Source: CAD feature listing. Evaluate the final solid. Frame: model axes, mm. Face numbers are marked on the shaded views. Round coordinates to 2 decimals unless told otherwise and drop trailing zeros. Write each loop counter-clockwise with the first axis right and the second up, starting at its lowest first coordinate (ties: lowest second). Pieces come first, ordered by that corner, then holes. Notation, with made-up numbers: M 89.25,0.25 L 126.25,0.25 A7 cw 126.25,4.25 Z; hole C 34,71.25 d10. An arc over 180 degrees is marked long. Answer in a Markdown table with one row per item.
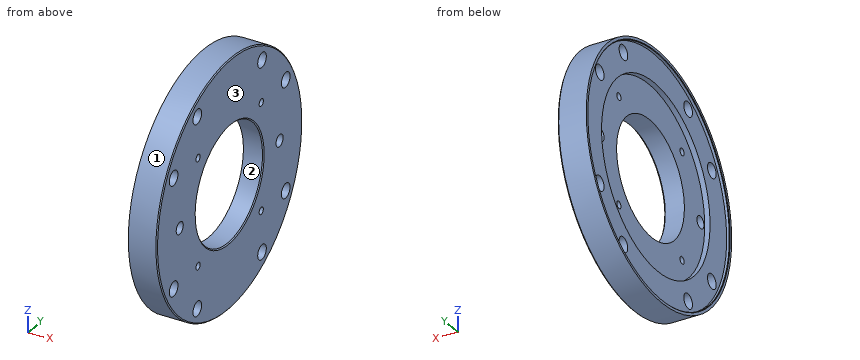
from build123d import *

# Parameters (mm, degrees)
CUT_EXTRUDE_1_DEPTH      = 170.04733065
CUT_EXTRUDE_1_DEPTH_BACK = 170.04733065
SKETCH_2_R               = 7
CUT_EXTRUDE_2_DEPTH      = 170.04733065
CUT_EXTRUDE_2_DEPTH_BACK = 170.04733065
SKETCH_3_R               = 3.4
CUT_EXTRUDE_3_DEPTH      = 170.04733065
CUT_EXTRUDE_3_DEPTH_BACK = 170.04733065
SKETCH_4_R               = 5.7225


with BuildPart() as part:
    # ｽｹｯﾁ1 → 回転1 (revolve)
    with BuildSketch(Plane.XY, mode=Mode.PRIVATE) as revolve_1_sk:
        Polygon((0, 117), (0, 56), (-1, 55), (-19, 55), (-19, 88), (-24, 88), (-24, 115), (-26.5, 115), (-27, 115.5), (-27, 118), (-1, 118), align=None)
    revolve(revolve_1_sk.sketch.rotate(Axis((-27, 0, 0), (1, 0, 0)), 90), axis=Axis((-27, 0, 0), (1, 0, 0)))

    # ｽｹｯﾁ2 → ｶｯﾄ - 押し出し1 (cut, two sides: drawn at the far end of the back side and taken through both)
    with BuildSketch(Plane(origin=(0, 0, 0), x_dir=(0, 0, -1), z_dir=(1, 0, 0)).offset(-CUT_EXTRUDE_1_DEPTH_BACK)):
        with Locations((90.932667397, 52.5)):
            Circle(SKETCH_2_R)
        with Locations((52.5, 90.932667397)):
            Circle(SKETCH_2_R)
        with Locations((-52.5, 90.932667397)):
            Circle(SKETCH_2_R)
        with Locations((-90.932667397, 52.5)):
            Circle(SKETCH_2_R)
        with Locations((-90.932667397, -52.5)):
            Circle(SKETCH_2_R)
        with Locations((-52.5, -90.932667397)):
            Circle(SKETCH_2_R)
        with Locations((52.5, -90.932667397)):
            Circle(SKETCH_2_R)
        with Locations((90.932667397, -52.5)):
            Circle(SKETCH_2_R)
    extrude(amount=CUT_EXTRUDE_1_DEPTH + CUT_EXTRUDE_1_DEPTH_BACK, mode=Mode.SUBTRACT)

    # ｽｹｯﾁ3 → ｶｯﾄ - 押し出し2 (cut, two sides: drawn at the far end of the back side and taken through both)
    with BuildSketch(Plane(origin=(0, 0, 0), x_dir=(0, 0, -1), z_dir=(1, 0, 0)).offset(-CUT_EXTRUDE_2_DEPTH_BACK)):
        with Locations((51.265241636, 51.265241636)):
            Circle(SKETCH_3_R)
        with Locations((-51.265241636, 51.265241636)):
            Circle(SKETCH_3_R)
        with Locations((-51.265241636, -51.265241636)):
            Circle(SKETCH_3_R)
        with Locations((51.265241636, -51.265241636)):
            Circle(SKETCH_3_R)
    extrude(amount=CUT_EXTRUDE_2_DEPTH + CUT_EXTRUDE_2_DEPTH_BACK, mode=Mode.SUBTRACT)

    # ｽｹｯﾁ4 → ｶｯﾄ - 押し出し3 (cut, two sides: drawn at the far end of the back side and taken through both)
    with BuildSketch(Plane(origin=(0, 0, 0), x_dir=(0, 0, -1), z_dir=(1, 0, 0)).offset(-CUT_EXTRUDE_3_DEPTH_BACK)):
        with Locations((0, 81)):
            Circle(SKETCH_4_R)
        with Locations((0, -81)):
            Circle(SKETCH_4_R)
    extrude(amount=CUT_EXTRUDE_3_DEPTH + CUT_EXTRUDE_3_DEPTH_BACK, mode=Mode.SUBTRACT)


solid = part.part
Q1. Section B-B (z = 0). State how many separate pieces and enclosed holes the cut face has, and give its area (3 significant figures).
Solutions:
| item | result |
|---|---|
| separate pieces | 4 |
| enclosed holes | 0 |
| area | 2,270 mm2 |
Q2. Pull-direction query (Z, two-part tool) for the marked faces 1, 2 and 3; classes: pulls with the +Z half, pulls with the -Z half, needs draft (parallel to the pull), parting line crosses it, or undercut.
Solutions:
| item | result |
|---|---|
| face 1 | parting line crosses it |
| face 2 | undercut |
| face 3 | needs draft |
Q3. Material intervals for probe 1 along Y at (x, z) = (-14.5, 0); probe 2 along Y at (x, z) = (-3.25, 49.5); probe 3 along Y at (x, z) = (-7, -95), sorted ascending.
Solutions:
| item | result |
|---|---|
| probe 1 | y = -118 to -86.72, -75.28 to -55, 55 to 75.28, 86.72 to 118 |
| probe 2 | y = -107.12 to -97.26, -84.61 to -54.17, -48.36 to -23.97, 23.97 to 48.36, 54.17 to 84.61, 97.26 to 107.12 |
| probe 3 | y = -69.99 to -58.2, -46.8 to 46.8, 58.2 to 69.99 |
Q4. Contact query for flat-ended pins moving along their axis: pin 1 Ø4 at (x, z) = (-23, -83.5) entering from -Y; pin 2 Ø5 at (x, y) = (-13, 41) entering from -Z; pin 3 Ø1.5 at (x, y) = (-17.5, -93) entering from +Z; pin 4 Ø10.5 at (y, z) = (-81, 0) entering from -X. Output: stop coordinate, or through.
Solutions:
| item | result |
|---|---|
| pin 1 | stops at y = -85.33 |
| pin 2 | stops at z = -111.54 |
| pin 3 | stops at z = 73.58 |
| pin 4 | passes through |
Q5. Section A-A (y = 0). Return loops of the section in (x, z).
Solutions:
| item | result |
|---|---|
| outline | M -27,-118 L -1,-118 L 0,-117 L 0,-56 L -1,-55 L -19,-55 L -19,-88 L -24,-88 L -24,-115 L -26.5,-115 L -27,-115.5 Z; M -27,115.5 L -26.5,115 L -24,115 L -24,88 L -19,88 L -19,55 L -1,55 L 0,56 L 0,117 L -1,118 L -27,118 Z |
